Build history of the part. All positions in model axes, mm. A direction names the side the tool comes from. Coordinates: 2 decimals unless noted, no trailing zeros. Write each loop counter-clockwise with the first axis right and the second up, starting at its lowest first coordinate (ties: lowest second). Pieces come first, ordered by that corner, then holes.
from build123d import *

# Parameters (mm, degrees)
SKETCH_1_R          = 1.1
SKETCH_1_R_2        = 1.6
EXTRUDE_1_DEPTH     = 3
SKETCH_2_R          = 1.6
SKETCH_2_R_2        = 1.1
EXTRUDE_2_DEPTH     = 3
SKETCH_3_W          = 16
SKETCH_3_H          = 36
EXTRUDE_3_DEPTH     = 30
FILLET_1_R          = 26
SKETCH_5_W          = 10
SKETCH_5_H          = 36
EXTRUDE_4_DEPTH     = 1
CUT_EXTRUDE_2_DEPTH = 36
SKETCH_6_R          = 0.85
SKETCH_6_R_2        = 10
CUT_EXTRUDE_1_DEPTH = 3
FILLET_2_R          = 0.5


with BuildPart() as part:
    # Sketch 1 → Extrude 1 (new body)
    with BuildSketch(Plane(origin=(0, 0, 0), x_dir=(1, 0, 0), z_dir=(0, 1, 0))):
        with BuildLine():
            Line((-8, 45), (-8, -13))
            Line((-8, -13), (8, -13))
            Line((8, -13), (8, 45))
            ThreePointArc((8, 45), (0, 53), (-8, 45))
        make_face()
        with Locations(Location((0, 51, 0), (0, 0, 270))):
            Circle(SKETCH_1_R, mode=Mode.SUBTRACT)
        with Locations(Location((4.242640687, 49.242640687, 0), (0, 0, 270))):
            Circle(SKETCH_1_R, mode=Mode.SUBTRACT)
        with Locations(Location((6, 45, 0), (0, 0, 270))):
            Circle(SKETCH_1_R, mode=Mode.SUBTRACT)
        with Locations(Location((4.242640687, 40.757359313, 0), (0, 0, 270))):
            Circle(SKETCH_1_R, mode=Mode.SUBTRACT)
        with Locations(Location((0, 39, 0), (0, 0, 270))):
            Circle(SKETCH_1_R, mode=Mode.SUBTRACT)
        with Locations(Location((-4.242640687, 40.757359313, 0), (0, 0, 270))):
            Circle(SKETCH_1_R, mode=Mode.SUBTRACT)
        with Locations(Location((-6, 45, 0), (0, 0, 270))):
            Circle(SKETCH_1_R, mode=Mode.SUBTRACT)
        with Locations(Location((-4.242640687, 49.242640687, 0), (0, 0, 270))):
            Circle(SKETCH_1_R, mode=Mode.SUBTRACT)
        with Locations(Location((0, 45, 0), (0, 0, 270))):
            Circle(SKETCH_1_R_2, mode=Mode.SUBTRACT)
    extrude(amount=EXTRUDE_1_DEPTH)



with BuildPart() as body_2:
    # Sketch 2 → Extrude 2 (new body)
    with BuildSketch(Plane(origin=(0, -36, 0), x_dir=(1, 0, 0), z_dir=(0, 1, 0))):
        with BuildLine():
            Line((8, -13), (8, 45))
            ThreePointArc((8, 45), (0, 53), (-8, 45))
            Line((-8, 45), (-8, -13))
            Line((-8, -13), (8, -13))
        make_face()
        with Locations(Location((0, 45, 0), (0, 0, 270))):
            Circle(SKETCH_2_R, mode=Mode.SUBTRACT)
        with Locations(Location((0, 51, 0), (0, 0, 270))):
            Circle(SKETCH_2_R_2, mode=Mode.SUBTRACT)
        with Locations(Location((4.242640687, 49.242640687, 0), (0, 0, 270))):
            Circle(SKETCH_2_R_2, mode=Mode.SUBTRACT)
        with Locations(Location((6, 45, 0), (0, 0, 270))):
            Circle(SKETCH_2_R_2, mode=Mode.SUBTRACT)
        with Locations(Location((4.242640687, 40.757359313, 0), (0, 0, 270))):
            Circle(SKETCH_2_R_2, mode=Mode.SUBTRACT)
        with Locations(Location((0, 39, 0), (0, 0, 270))):
            Circle(SKETCH_2_R_2, mode=Mode.SUBTRACT)
        with Locations(Location((-4.242640687, 40.757359313, 0), (0, 0, 270))):
            Circle(SKETCH_2_R_2, mode=Mode.SUBTRACT)
        with Locations(Location((-6, 45, 0), (0, 0, 270))):
            Circle(SKETCH_2_R_2, mode=Mode.SUBTRACT)
        with Locations(Location((-4.242640687, 49.242640687, 0), (0, 0, 270))):
            Circle(SKETCH_2_R_2, mode=Mode.SUBTRACT)
    extrude(amount=-EXTRUDE_2_DEPTH)


with BuildPart() as part_1:
    add(part.part)

    add(body_2.part)  # Extrude 3 merges body 2
    # Sketch 3 → Extrude 3 (add)
    with BuildSketch(Plane.XY.offset(13)):
        with Locations((0, -18)):
            Rectangle(SKETCH_3_W, SKETCH_3_H)
    extrude(amount=-EXTRUDE_3_DEPTH)

    # Fillet 1
    # the kernel refuses this fillet: 26 mm, written as the material it takes off along each edge
    with BuildSketch(Plane(origin=(-8, -99, 13), x_dir=(0, 0, -1), z_dir=(0, 1, 0))) as fillet_1_piece_1:
        with BuildLine():
            CenterArc((24, -26), FILLET_1_R, 90, 67.380135052)
            Line((0, -16), (-0.48, -15.8))
            ThreePointArc((-0.48, -15.8), (-0.52, -8), (-0.52, 0))
            Line((-0.52, 0), (0, 0.52))
            Line((0, 0.52), (24, 0.52))
            Line((24, 0.52), (24, 0))
        make_face()
    extrude(amount=162, mode=Mode.SUBTRACT)

    # Sketch 5 → Extrude 4 (add)
    with BuildSketch(Plane.ZY.offset(8)):
        with Locations((-22, -18)):
            Rectangle(SKETCH_5_W, SKETCH_5_H)
    extrude(amount=-EXTRUDE_4_DEPTH)

    # Sketch 7 → Cut-Extrude 2 (cut)
    with BuildSketch(Plane.XZ):
        with BuildLine():
            Line((5, 7.973665961), (5, -17))
            Line((5, -17), (-5, -17))
            Line((-5, -17), (-5, -11))
            ThreePointArc((-5, -11), (-2.346989949, -0.276194705), (5, 7.973665961))
        make_face()
    extrude(amount=CUT_EXTRUDE_2_DEPTH, mode=Mode.SUBTRACT)

    # Sketch 6 → Cut-Extrude 1 (cut)
    with BuildSketch(Plane(origin=(8, 0, 0), x_dir=(0, 0, -1), z_dir=(1, 0, 0))):
        with Locations((11, -6.631182999)):
            Circle(SKETCH_6_R)
        with Locations((-7, -6.631182999)):
            Circle(SKETCH_6_R)
        with Locations((-7, -29.368817001)):
            Circle(SKETCH_6_R)
        with Locations((11, -29.368817001)):
            Circle(SKETCH_6_R)
        with Locations((2, -18)):
            Circle(SKETCH_6_R_2)
    extrude(amount=-CUT_EXTRUDE_1_DEPTH, mode=Mode.SUBTRACT)

    # Fillet 2
    fillet_2_edges = [part_1.edges().sort_by_distance(p)[0] for p in [
        (8, -18, 13),
    ]]
    fillet(fillet_2_edges, radius=FILLET_2_R)


solid = part_1.part
(1) Two-plate mould, pull along X, no slides. Class faces 1 (the cylindrical face through (6.521, -30.123, 6.608)), 2 (the cylindrical face through (4.573, -37.479, -48.193)), 3 (the flat face through (0, -36, -30)), 4 (the cylindrical face through (0, -37, -53)): pulls with the +X half, pulls with the -X half, needs draft (parallel to the pull), parting line crosses it, or undercut.
(2) Slice it at B-B, the plane z = -39. List the corners of the cut face in (x, y).
(3) Probe L1, parallel to Y at x = 2.5, z = -17.5; L2, parallel to Y at x = 7.25, z = -11; L3, parallel to X at y = -13, z = -11. List the from-to ranges inside material, lowest first.
(4) Slice it at C-C, the plane z = -16. List the corners of the cut face in (x, y), and give its area (3 significant figures).
(5) Flat gauge pins, fed straight in: P1, Ø3, axis at x = -5, y = -4, coming from the +Z side; P2, Ø2, axis at x = -6.5, y = -11, coming from the -Z side; P3, Ø6, axis at x = 5, y = -26.5, coming from the -Z side. Where does each tip first touch, or does it go through?
(6) Slice it at D-D, the plane x = 6. List the corners of the cut face in (y, z), and give its area (3 significant figures).
(7) 3-axis set-ups, long thin cutter, end or side, ignore diameter. For faces 5 (the cylindrical face through (0.33, 1.48, -37.95)), 6 (the flat face through (6, -18, -17)), 7 (the cylindrical face through (6.521, -7.385, 6.608)): which of +Z, -Z, +X, -X, +Y, -Y reach the whole face in a straight line?
Results:
1. face 1: needs draft
1. face 2: undercut
1. face 3: undercut
1. face 4: parting line crosses it
2. outline: (-8, -39) - (-1.1, -39) - (-1.1, -36) - (-8, -36) - close; (-8, 0) - (-1.1, 0) - (-1.1, 3) - (-8, 3) - close; (1.1, -39) - (8, -39) - (8, -36) - (1.1, -36) - close; (1.1, 0) - (8, 0) - (8, 3) - (1.1, 3) - close
3. L1: y = -39 to -36, 0 to 3
3. L2: y = -39 to -30.22, -28.52 to -22.36, -13.64 to -7.48, -5.78 to 3
3. L3: x = -8 to -5, 5 to 8
4. outline: (-8, -39) - (8, -39) - (8, 3) - (-8, 3) - close; hole (-5, -36) - (5, -36) - (5, 0) - (-5, 0) - close
4. area: 312 mm2
5. P1: stops at z = 3.62
5. P2: stops at z = -27
5. P3: stops at z = -17
6. outline: (-39, -50.29) - (-36, -50.29) - (-36, -46.1) - (-39, -46.1) - close; (-39, -43.9) - (-36, -43.9) - (-36, -17) - (0, -17) - (0, -43.9) - (3, -43.9) - (3, 12.07) - (-39, 12.07) - close; (0, -50.29) - (3, -50.29) - (3, -46.1) - (0, -46.1) - close; hole circle Ø1.7 at (-29.37, -11); hole circle Ø1.7 at (-29.37, 7); hole circle Ø20 at (-18, -2); hole circle Ø1.7 at (-6.63, -11); hole circle Ø1.7 at (-6.63, 7)
6. area: 1,080 mm2
7. face 5: +Y, -Y
7. face 6: -Z, +X
7. face 7: +X
